```python
from build123d import *

# Parameters (mm, degrees)
CROQUIS1_R              = 2.1
SALIENTE_EXTRUIR1_DEPTH = 6
SALIENTE_EXTRUIR3_DEPTH = 1
REDONDEO2_R             = 1
SALIENTE_EXTRUIR5_DEPTH = 6


with BuildPart() as part:
    # Croquis1 → Saliente-Extruir1 (new body)
    with BuildSketch(Plane.XY):
        with BuildLine():
            ThreePointArc((-114.035873061, -9.790567955), (-34.858360528, -14.975714339), (42.681169488, 1.864283248))
            ThreePointArc((42.681169488, 1.864283248), (48.601198063, 14.707696411), (35.7577849, 20.627724986))
            ThreePointArc((35.7577849, 20.627724986), (-36.341639472, 4.969206908), (-109.964126939, 9.790567955))
            ThreePointArc((-109.964126939, 9.790567955), (-121.790567955, 2.035873061), (-114.035873061, -9.790567955))
        make_face()
        with Locations((-112, 0)):
            Circle(CROQUIS1_R, mode=Mode.SUBTRACT)
        with Locations((39.219477194, 11.246004117)):
            Circle(CROQUIS1_R, mode=Mode.SUBTRACT)
        Circle(CROQUIS1_R, mode=Mode.SUBTRACT)
        with BuildLine():
            ThreePointArc((-18.792854848, -10.296017287), (-12.777386897, -2.433820054), (-20.63958413, 3.581647897))
            ThreePointArc((-20.63958413, 3.581647897), (-56, 1.239230948), (-91.36041587, 3.581647897))
            ThreePointArc((-91.36041587, 3.581647897), (-99.222613103, -2.433820054), (-93.207145152, -10.296017287))
            ThreePointArc((-93.207145152, -10.296017287), (-56, -12.760769052), (-18.792854848, -10.296017287))
        make_face(mode=Mode.SUBTRACT)
    extrude(amount=SALIENTE_EXTRUIR1_DEPTH)

    # Croquis3 → Saliente-Extruir3 (add, symmetric)
    with BuildSketch(Plane.XY.offset(3)):
        with BuildLine():
            ThreePointArc((-98.228577232, -7.053046158), (-96.081427883, -9.237480134), (-93.207145152, -10.296017287))
            ThreePointArc((-93.207145152, -10.296017287), (-56, -12.760769052), (-18.792854848, -10.296017287))
            ThreePointArc((-18.792854848, -10.296017287), (-15.918572117, -9.237480134), (-13.771422768, -7.053046158))
            ThreePointArc((-13.771422768, -7.053046158), (-56, -10.260769052), (-98.228577232, -7.053046158))
        make_face()
        with BuildLine():
            ThreePointArc((-98.228577232, 7.624636675), (-56, 6.557109307), (-13.771422768, 7.624636675))
            ThreePointArc((-13.771422768, 7.624636675), (-56, 4.239230948), (-98.228577232, 7.624636675))
        make_face()
    extrude(amount=SALIENTE_EXTRUIR3_DEPTH, both=True)

    # Redondeo2
    redondeo2_edges = [part.edges().sort_by_distance(p)[0] for p in [
        (-96.081427883, -9.237480134, 2),
        (-56, -12.760769052, 2),
        (-15.918572117, -9.237480134, 2),
        (-96.081427883, -9.237480134, 4),
        (-56, -12.760769052, 4),
        (-15.918572117, -9.237480134, 4),
        (-56, 4.239230948, 2),
        (-56, 4.239230948, 4),
    ]]
    fillet(redondeo2_edges, radius=REDONDEO2_R)

    # Croquis1<3> → Saliente-Extruir5 (add)
    with BuildSketch(Plane.XY):
        with BuildLine():
            ThreePointArc((-121.405666345, -8.258076308), (-129.160361239, 3.568364708), (-117.333920224, 11.323059602))
            Line((-117.333920224, 11.323059602), (-109.964126939, 9.790567955))
            ThreePointArc((-109.964126939, 9.790567955), (-121.790567955, 2.035873061), (-114.035873061, -9.790567955))
            Line((-114.035873061, -9.790567955), (-121.405666345, -8.258076308))
        make_face()
    extrude(amount=SALIENTE_EXTRUIR5_DEPTH)


solid = part.part
```
Could you check a few things on this model? Use its own coordinates, in mm. A direction names the side the tool comes from. Give positions to 0.01 mm unless a question says otherwise; leave off trailing zeros. Order: outer loops, then holes, each group sorted by start corner. A loop starts at its lowest first (then second) coordinate and runs counter-clockwise, first axis right, second up.
Q1. Suppose I cut it at C-C, the plane x = -107. Write out the boundary of the cut face in (y, z), and give its area (3 significant figures).
Q2. We'd pull the mould along X, two halves only. Please class faces 1 (the flat face through (-117.669, -9.035, 2.958)), 2 (the cylindrical face through (-35.97, -15.056, 2.958)), 3 (the cylindrical face through (-18.96, 6.84, 0.29)), 4 (the flat face through (-33, 4, 0)): +X half, -X half, draft (parallel to the pull), parting line (faces both ways), or undercut.
Q3. Suppose I cut it at B-B, the plane x = 0. Write out the boundary of the cut face in (y, z), and give its area (3 significant figures).
Q4. For faces 5 (the flat face through (-56, -11, 2)), 6 (the cylindrical face through (-55.5, 1.24, 2.96)), 7 (the flat face through (-56, -11, 4)), 8 (the flat face through (-113.701, 10.568, 2.958)), 9 (the flat face through (-33, 4, 6)), which set-ups out of +Z, -Z, +X, -X, +Y, -Y let a thin tool reach every point of the face, with its end or its side?
Q5. I'm going to push flat-ended pins straight in: P1, Ø4, axis at x = -75.5, y = -7, coming from the +Z side; P2, Ø1.5, axis at x = -53.5, y = 5.5, coming from the +Z side; P3, Ø5, axis at x = -47, y = -9.5, coming from the -Z side; P4, Ø3.5, axis at x = -45.5, y = -9.5, coming from the +Z side. Where does each tip first touch, or does it pass through?
Q6. If I drill on line 1 along Y through (x, z) = (-56.5, 5.5); line 2 along Y through (x, z) = (-57, 3.25); line 3 along Y through (x, z) = (21, 4), over which ranges is the centre line in solid material (lowest first)?
Q7. Suppose I cut it at A-A, the plane y = -5. Write out the boundary of the cut face in (x, z), and give its area (3 significant figures).
Solution:
1. outline: (-11.16, 0) - (9.19, 0) - (9.19, 6) - (-11.16, 6) - close
1. area: 122 mm2
2. face 1: -X half
2. face 2: parting line
2. face 3: undercut
2. face 4: draft
3. outline: (-10.21, 0) - (-2.1, 0) - (-2.1, 6) - (-10.21, 6) - close; (2.1, 0) - (10.22, 0) - (10.22, 6) - (2.1, 6) - close
3. area: 97.4 mm2
4. face 5: -Z
4. face 6: +Z, -Z
4. face 7: +Z
4. face 8: +Z, -Z, +Y
4. face 9: +Z, +X, -X, +Y, -Y
5. P1: passes through
5. P2: stops at z = 4.13
5. P3: stops at z = 1.92
5. P4: stops at z = 4
6. line 1: y = -15.76 to -12.76, 1.24 to 4.24
6. line 2: y = -15.76 to -10.26, 1.24 to 6.56
6. line 3: y = -5.16 to 15.67
7. outline: (-126.94, 0) - (-99.09, 0) - (-99.09, 6) - (-126.94, 6) - close; (-12.91, 0) - (21.58, 0) - (21.58, 6) - (-12.91, 6) - close
7. area: 374 mm2
